from build123d import *

# Parameters (mm, degrees)
SKETCH_1_W      = 590
SKETCH_1_H      = 30
SKETCH_1_R      = 5
EXTRUDE_1_DEPTH = 5
FILLET_1_R      = 10
FILLET_2_R      = 1


with BuildPart() as part:
    # 스케치1 → 보스-돌출1 (new body)
    with BuildSketch(Plane.XY):
        with Locations((5.677604278, 40.167322835)):
            Rectangle(SKETCH_1_W, SKETCH_1_H)
        with Locations((-279.322395722, 40.167322835)):
            Circle(SKETCH_1_R, mode=Mode.SUBTRACT)
        with Locations((290.677604278, 40.167322835)):
            Circle(SKETCH_1_R, mode=Mode.SUBTRACT)
        with Locations((5.677604278, 40.167322835)):
            Circle(SKETCH_1_R, mode=Mode.SUBTRACT)
    extrude(amount=EXTRUDE_1_DEPTH)

    # 필렛1
    fillet_1_edges = [part.edges().sort_by_distance(p)[0] for p in [
        (-289.322395722, 55.167322835, 2.5),
        (300.677604278, 55.167322835, 2.5),
        (300.677604278, 25.167322835, 2.5),
        (-289.322395722, 25.167322835, 2.5),
    ]]
    fillet(fillet_1_edges, radius=FILLET_1_R)

    # 필렛2
    fillet_2_edges = [part.edges().sort_by_distance(p)[0] for p in [
        (300.677604278, 40.167322835, 0),
        (300.677604278, 40.167322835, 5),
        (-289.322395722, 40.167322835, 0),
        (5.677604278, 55.167322835, 0),
        (5.677604278, 25.167322835, 0),
        (-286.393463534, 52.238390647, 0),
        (-286.393463534, 28.096255023, 0),
        (297.748672089, 52.238390647, 0),
        (297.748672089, 28.096255023, 0),
        (5.677604278, 25.167322835, 5),
        (-289.322395722, 40.167322835, 5),
        (5.677604278, 55.167322835, 5),
        (-286.393463534, 52.238390647, 5),
        (-286.393463534, 28.096255023, 5),
        (297.748672089, 52.238390647, 5),
        (297.748672089, 28.096255023, 5),
    ]]
    fillet(fillet_2_edges, radius=FILLET_2_R)


solid = part.part
CAD build for the part. Positions are in the model's coordinates, mm. Give positions to 0.01 mm unless a question says otherwise; leave off trailing zeros. Loops run counter-clockwise (first coordinate to the right, second up) from the corner with the lowest first, then second, coordinate; pieces in that order, holes last. Notation, with made-up numbers: M 10,-6 L 68,-6 A30 cw 68,27 Z; hole C -2,-30.75 d1. An arc over 180 degrees is marked long. Answer in a Markdown table with one row per item. Add a question column.
Item 1: Mould opens along X. For faces 1 (the face through (297.67, 28.02, 2.52)), 2 (the face through (-284.318, 40.387, 2.465)), 3 (the face through (285.682, 40.387, 2.465)), 4 (the face through (1.6, 43.5, 5)) say: +X half, -X half, draft (parallel to the pull), parting line (faces both ways), or undercut.
Item 2: Band-saw the part on A-A on z = 2.6. Give the cut face in (x, y).
Item 3: Probe probe 1 along X at (y, z) = (40, 0.65); probe 2 along X at (y, z) = (37, 2.9); probe 3 along Z at (x, y) = (-122.5, 26). List the from-to ranges inside material, lowest first.
Item 4: Drop flat-ended pins along their axis: P1, Ø4, axis at x = -212.5, y = 33, coming from the -Z side; P2, Ø1, axis at y = 34.5, z = 3, coming from the +X side. Give the stop position or say it passes through.
Reply:
| question | item | result |
|---|---|---|
| 1 | face 1 | +X half |
| 1 | face 2 | undercut |
| 1 | face 3 | undercut |
| 1 | face 4 | draft |
| 2 | outline | M -289.32,35.17 A10 ccw -279.32,25.17 L 290.68,25.17 A10 ccw 300.68,35.17 L 300.68,45.17 A10 ccw 290.68,55.17 L -279.32,55.17 A10 ccw -289.32,45.17 Z; hole C -279.32,40.17 d10; hole C 5.68,40.17 d10; hole C 290.68,40.17 d10 |
| 3 | probe 1 | x = -289.26 to -284.32, -274.33 to 0.68, 10.67 to 285.68, 295.67 to 300.61 |
| 3 | probe 2 | x = -289.32 to -283.19, -275.45 to 1.81, 9.55 to 286.81, 294.55 to 300.68 |
| 3 | probe 3 | z = 0.01 to 4.99 |
| 4 | P1 | stops at z = 0 |
| 4 | P2 | stops at x = 300.68 |
